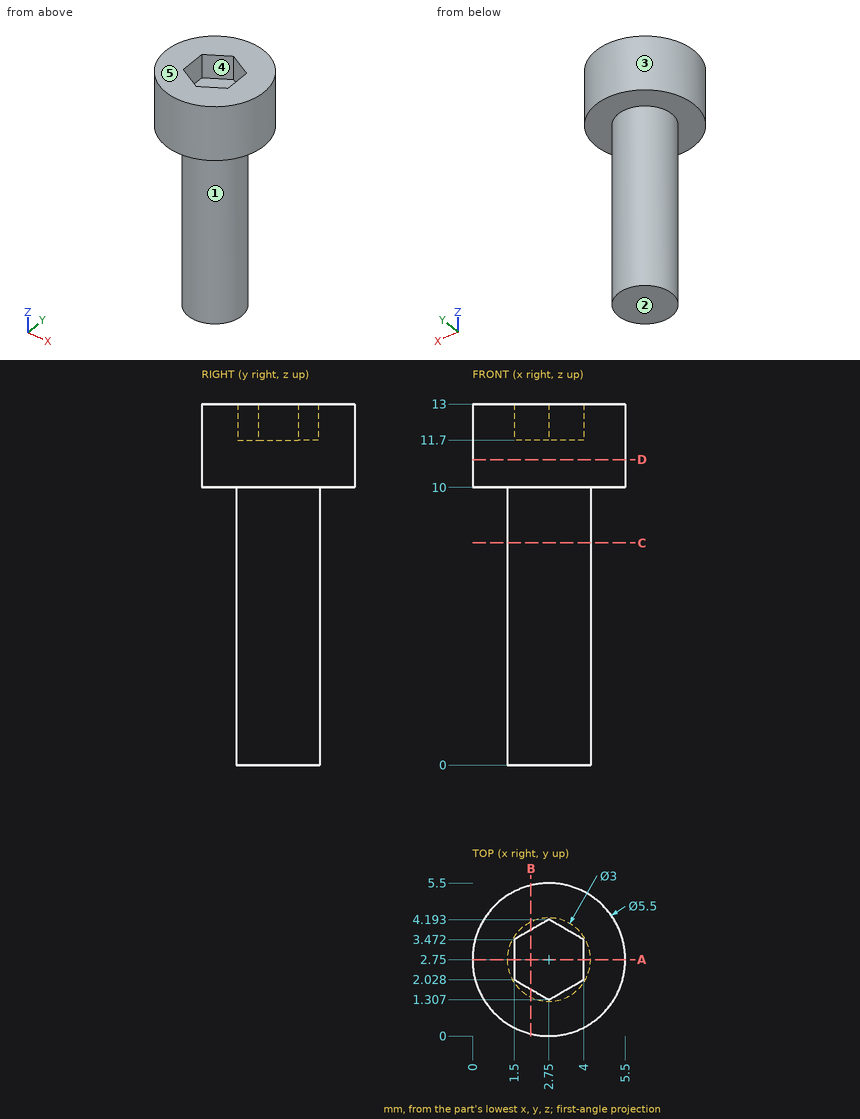
Job drawing, mm, ordinate dimensions from the low corner. One solid piece. A direction names the side the tool comes from. Give positions to 0.01 mm unless a question says otherwise; leave off trailing zeros. Loops run counter-clockwise (first coordinate to the right, second up) from the corner with the lowest first, then second, coordinate; pieces in that order, holes last. Notation, with made-up numbers: M 84.5,-18 L 131.5,-18 A26 ccw 131.5,13 Z; hole C -39.75,-35 d9. An arc over 180 degrees is marked long. Answer in a Markdown table with one row per item. Add a question column.
Item 1: Band-saw the part on D-D on z = 11. Give the cut face in (x, y).
Item 2: Drop flat-ended pins along their axis: P1, Ø1.5, axis at x = 4.5, z = 5.5, coming from the +Y side; P2, Ø1, axis at y = 2.5, z = 8.5, coming from the +X side; P3, Ø3, axis at x = 2.5, y = 2.5, coming from the +Z side; P4, Ø1.5, axis at y = 2.5, z = 5, coming from the -X side. Give the stop position or say it passes through.
Item 3: Band-saw the part on A-A on y = 2.75. Give the cut face in (x, z).
Item 4: Tool access for the marked faces 1 and 2: list every direction of +Z, -Z, +X, -X, +Y, -Y with a clear straight run to the whole face (end or side of a thin tool).
Item 5: Band-saw the part on C-C on z = 8. Give the cut face in (x, y).
Item 6: Band-saw the part on B-B on x = 2.1. Give the cut face in (y, z), then the cut area to 3 significant figures.
Item 7: Mould opens along Y. For the marked faces 3, 4 and 5 say: +Y half, -Y half, draft (parallel to the pull), parting line (faces both ways), or undercut.
Item 8: Probe probe 1 along Z at (x, y) = (3.35, 2.35); probe 2 along Z at (x, y) = (3.9, 5.1); probe 3 along Y at (x, z) = (2.35, 5.75) (1 decimal). List the from-to ranges inside material, lowest first.
Reply:
| question | item | result |
|---|---|---|
| 1 | outline | C 2.75,2.75 d5.5 |
| 2 | P1 | stops at y = 3.87 |
| 2 | P2 | stops at x = 4.25 |
| 2 | P3 | stops at z = 13 |
| 2 | P4 | stops at x = 1.25 |
| 3 | outline | M 0,10 L 1.25,10 L 1.25,0 L 4.25,0 L 4.25,10 L 5.5,10 L 5.5,13 L 4,13 L 4,11.7 L 1.5,11.7 L 1.5,13 L 0,13 Z |
| 4 | face 1 | -Z |
| 4 | face 2 | -Z, +X, -X, +Y, -Y |
| 5 | outline | C 2.75,2.75 d3 |
| 6 | outline | M 0.08,10 L 1.4,10 L 1.4,0 L 4.1,0 L 4.1,10 L 5.42,10 L 5.42,13 L 3.82,13 L 3.82,11.7 L 1.68,11.7 L 1.68,13 L 0.08,13 Z |
| 6 | area | 40.3 mm^2 |
| 7 | face 3 | parting line |
| 7 | face 4 | undercut |
| 7 | face 5 | draft |
| 8 | probe 1 | z = 0 to 11.7 |
| 8 | probe 2 | z = 10 to 13 |
| 8 | probe 3 | y = 1.3 to 4.2 |
